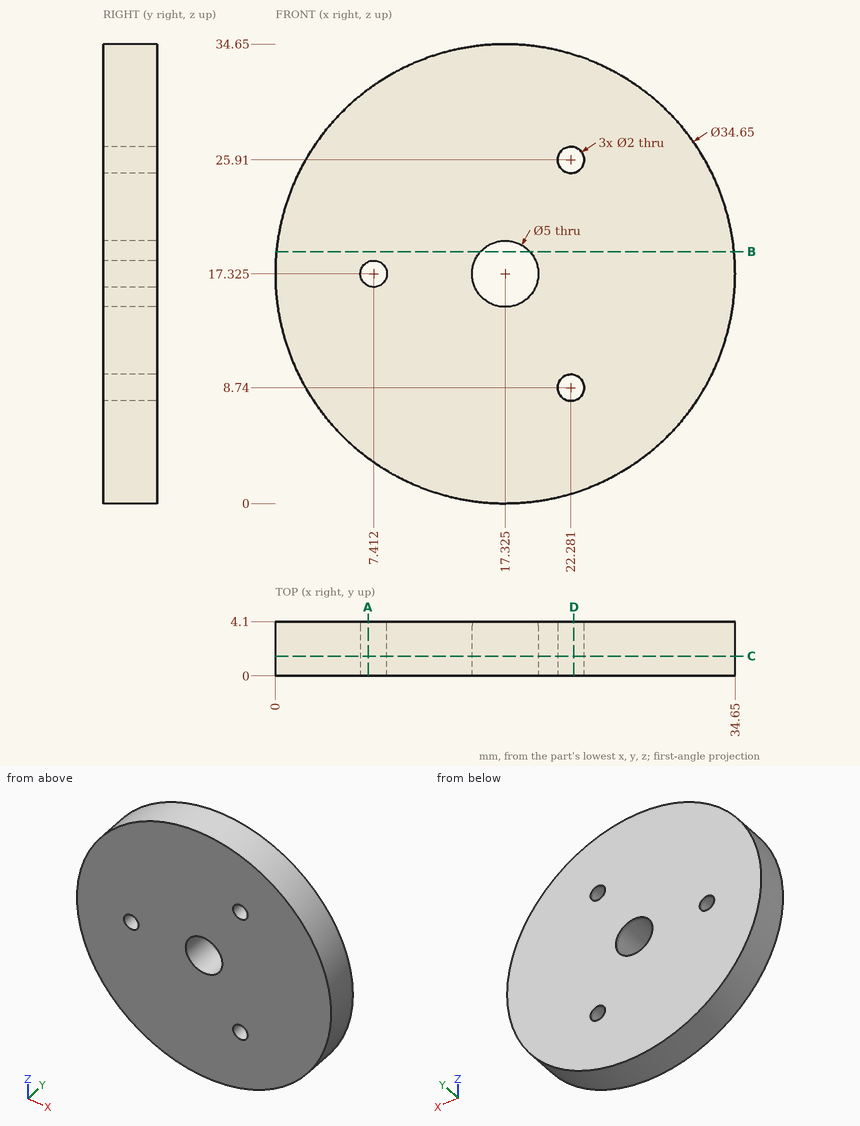
Geometry: see drawing. Coordinates: mm, zero at the bounding-box minimum. Round coordinates to 2 decimals unless told otherwise and drop trailing zeros. Loops run counter-clockwise (first coordinate to the right, second up) from the corner with the lowest first, then second, coordinate; pieces in that order, holes last. Notation, with made-up numbers: (13.5, -34) - (54.5, -34) arc R26 cw to (54.5, -6) - close; hole circle Ø1 at (39, 63.25). An arc over 180 degrees is marked (long way). Use CSV: the item, a comma, the result in double quotes.
Q1. Section query B-B, the plane z = 19. Output: boundary loops of the cut face in (x, y), then the cut area to 3 significant figures.
Reported:
outline,"(0.08, 0) - (15.47, 0) - (15.47, 4.1) - (0.08, 4.1) - close; (19.18, 0) - (34.57, 0) - (34.57, 4.1) - (19.18, 4.1) - close"
area,"126 mm^2"
Q2. Section query A-A, the plane x = 7. Output: boundary loops of the cut face in (y, z) (1 decimal).
Reported:
outline,"(0, 3.4) - (4.1, 3.4) - (4.1, 16.4) - (0, 16.4) - close; (0, 18.2) - (4.1, 18.2) - (4.1, 31.2) - (0, 31.2) - close"
Q3. Ray query, line 1 along Z through (x, y) = (21.5, 0.7) (1 decimal); line 2 along Z through (x, y) = (22.5, 3.3) (1 decimal); line 3 along X through (y, z) = (2.65, 8) (1 decimal). Return the intervals inside material, ascending.
Reported:
line 1,"0.5 to 8.1, 9.4 to 25.3, 26.5 to 34.1"
line 2,"0.8 to 7.8, 9.7 to 24.9, 26.9 to 33.9"
line 3,"2.7 to 21.6, 23 to 31.9"
Q4. Section query D-D, the plane x = 22.5. Output: boundary loops of the cut face in (y, z) (1 decimal).
Reported:
outline,"(0, 0.8) - (4.1, 0.8) - (4.1, 7.8) - (0, 7.8) - close; (0, 9.7) - (4.1, 9.7) - (4.1, 24.9) - (0, 24.9) - close; (0, 26.9) - (4.1, 26.9) - (4.1, 33.9) - (0, 33.9) - close"
Q5. Section query C-C, the plane y = 1.5. Give the number of separate pieces and of enclosed holes in the cut face, then the cut area to 3 significant figures.
Reported:
separate pieces,"1"
enclosed holes,"4"
area,"914 mm^2"
Q6. Pin query (flat end, axial travel): pin 1 Ø8 at (x, z) = (17.325, 17.325) entering from -Y; pin 2 Ø1.2 at (x, z) = (7.41, 17.32) entering from -Y. Return the tip coordinate at first contact, or that it passes through.
Reported:
pin 1,"y = 0"
pin 2,"through"
